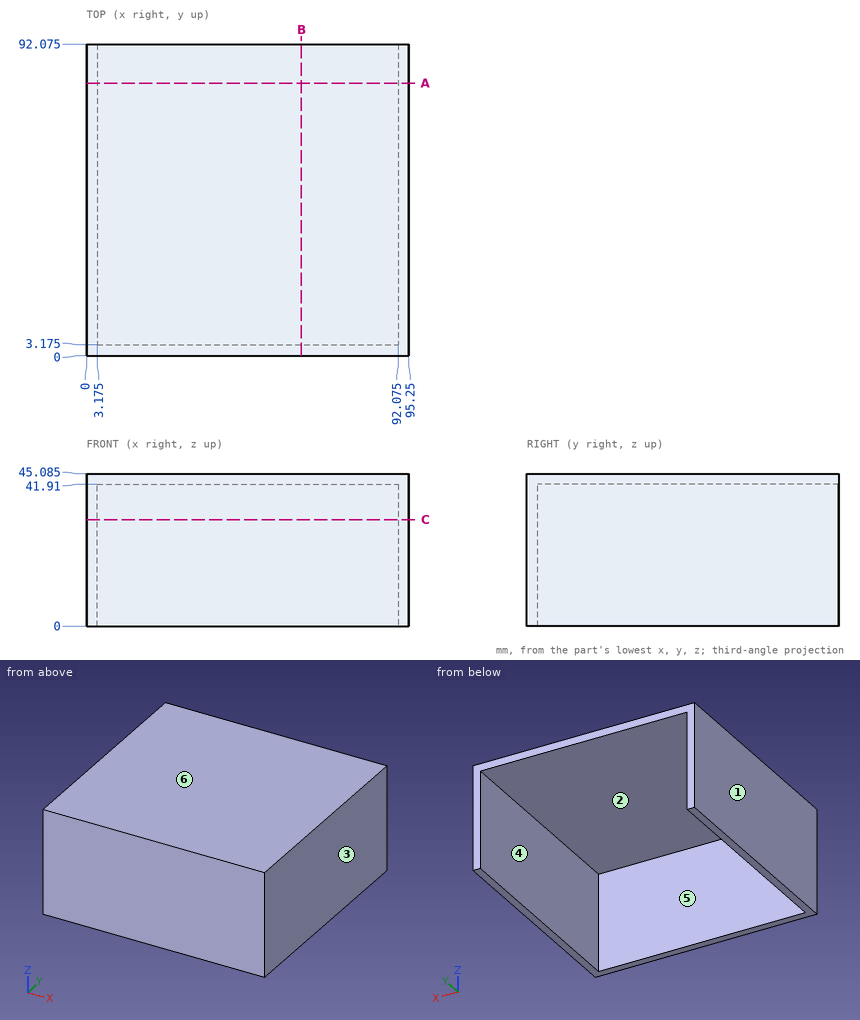
For this review, use the dimensioned drawing (mm, ordinates from the lowest corner) and the shaded views. A direction names the side the tool comes from. Coordinates: 2 decimals unless noted, no trailing zeros. Write each loop counter-clockwise with the first axis right and the second up, starting at its lowest first coordinate (ties: lowest second). Pieces come first, ordered by that corner, then holes. Notation, with made-up numbers: (64.25, 88) - (90.25, 88) arc R24 ccw to (90.25, 119) - close; hole circle Ø10 at (-23, 60.5). An arc over 180 degrees is marked (long way). Answer in a Markdown table with one row per item. Add a question column.
Q1. Consider section C-C on z = 31.5. Give the boundary of the cut face in (x, y) (3 decimals).
Q2. To check wall thickness, follow line 1 along X through (y, z) = (75, 31.5) (3 decimals); line 2 along Y through (x, z) = (7.5, 41.5) (3 decimals); line 3 along Z through (x, y) = (73.5, 5) (3 decimals). State the ranges of each line that lie inside material, in increasing order. Write a range as from..to.
Q3. Consider section A-A on y = 80.5. Give the boundary of the cut face in (x, z) (3 decimals).
Q4. For the marked faces 5 and 6, list the 3-axis set-ups (+Z, -Z, +X, -X, +Y, -Y) from which the entire face can be reached by the end or side of a thin tool; tool diameter is ignored.
Q5. Clearance check with flat-ended pins moving along their axes: pin 1 (12 mm diameter, centred on x = 33, y = 56.5, fed in from -Z); pin 2 (8 mm diameter, centred on x = 77, z = 26.5, fed in from +Y) (3 decimals). State where each tip first meets the part, or that it passes through.
Q6. Draft analysis for pull direction X (two halves, no side actions). For the marked faces 1, 2, 3 and 4, state which applies: +X half, -X half, draft (parallel to the pull), parting line (faces both ways), or undercut.
Q7. Consider section B-B on x = 63.5. Give the boundary of the cut face in (y, z) (3 decimals), then the cut area to 3 significant figures.
Answers below:
| question | item | result |
|---|---|---|
| 1 | outline | (0, 0) - (95.25, 0) - (95.25, 92.075) - (92.075, 92.075) - (92.075, 3.175) - (3.175, 3.175) - (3.175, 92.075) - (0, 92.075) - close |
| 2 | line 1 | 0..3.175, 92.075..95.25 |
| 2 | line 2 | 0..3.175 |
| 2 | line 3 | 41.91..45.085 |
| 3 | outline | (0, 0) - (3.175, 0) - (3.175, 41.91) - (92.075, 41.91) - (92.075, 0) - (95.25, 0) - (95.25, 45.085) - (0, 45.085) - close |
| 4 | face 5 | -Z, +Y |
| 4 | face 6 | +Z, +X, -X, +Y, -Y |
| 5 | pin 1 | z = 41.91 |
| 5 | pin 2 | y = 3.175 |
| 6 | face 1 | -X half |
| 6 | face 2 | undercut |
| 6 | face 3 | +X half |
| 6 | face 4 | undercut |
| 7 | outline | (0, 0) - (3.175, 0) - (3.175, 41.91) - (92.075, 41.91) - (92.075, 45.085) - (0, 45.085) - close |
| 7 | area | 425 mm² |
